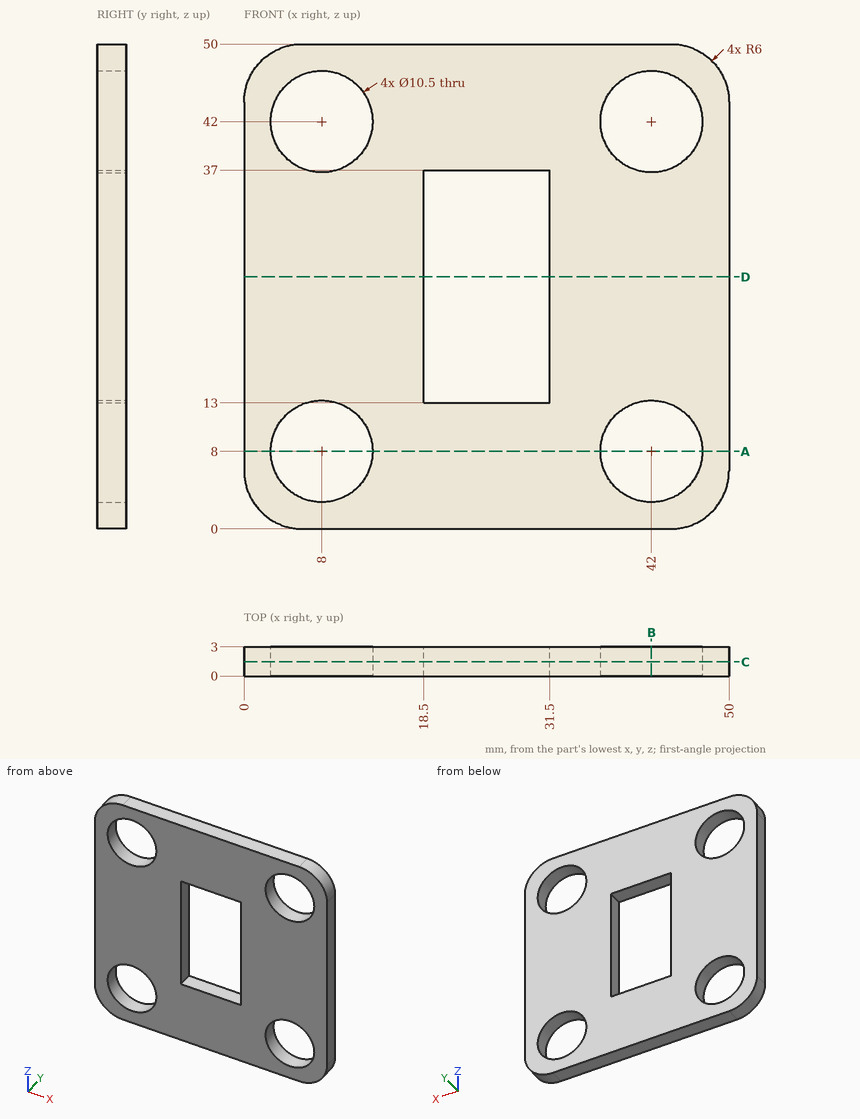
The figure shows three views and two pictorial views of one solid part (mm, origin at its lowest corner). Answer the questions. Round coordinates to 2 decimals unless told otherwise and drop trailing zeros. Write each loop counter-clockwise with the first axis right and the second up, starting at its lowest first coordinate (ties: lowest second). Pieces come first, ordered by that corner, then holes. Notation, with made-up numbers: (81, 56) - (115, 56) arc R32 ccw to (115, 86) - close; hole circle Ø11 at (8, 61.25). An arc over 180 degrees is marked (long way). Use one line per item in the form item = value. Start each with the question number.
Item 1: A cutting plane is placed at A-A (z = 8). Write down the section's boundary in (x, y), plus the area to 3 significant figures.
Item 2: Find the intervals of material crossed by line 1 (X direction, y = 1.1, z = 8); line 2 (Z direction, x = 44, y = 1.35), in increasing order. Write a range as [from, to].
Item 3: A cutting plane is placed at B-B (x = 42). Write down the section's boundary in (y, z).
Item 4: A cutting plane is placed at D-D (z = 26). Write down the section's boundary in (x, y).
Item 5: A cutting plane is placed at C-C (y = 1.45). Write down the section's boundary in (x, z).
The answers:
q1.outline = (0, 0) - (2.75, 0) - (2.75, 3) - (0, 3) - close; (13.25, 0) - (36.75, 0) - (36.75, 3) - (13.25, 3) - close; (47.25, 0) - (50, 0) - (50, 3) - (47.25, 3) - close
q1.area = 87.0 mm^2
q2.line_1 = [0, 2.75], [13.25, 36.75], [47.25, 50]
q2.line_2 = [0, 3.15], [12.85, 37.15], [46.85, 50]
q3.outline = (0, 0) - (3, 0) - (3, 2.75) - (0, 2.75) - close; (0, 13.25) - (3, 13.25) - (3, 36.75) - (0, 36.75) - close; (0, 47.25) - (3, 47.25) - (3, 50) - (0, 50) - close
q4.outline = (0, 0) - (18.5, 0) - (18.5, 3) - (0, 3) - close; (31.5, 0) - (50, 0) - (50, 3) - (31.5, 3) - close
q5.outline = (0, 6) arc R6 ccw to (6, 0) - (44, 0) arc R6 ccw to (50, 6) - (50, 44) arc R6 ccw to (44, 50) - (6, 50) arc R6 ccw to (0, 44) - close; hole circle Ø10.5 at (8, 8); hole circle Ø10.5 at (8, 42); hole (18.5, 13) - (31.5, 13) - (31.5, 37) - (18.5, 37) - close; hole circle Ø10.5 at (42, 8); hole circle Ø10.5 at (42, 42)
